from build123d import *

# Parameters (mm, degrees)
SKETCH1_W                                           = 20
SKETCH1_H                                           = 30
BOSS_EXTRUDE1_DEPTH                                 = 3
CSK_FOR_M3_COUNTERSUNK_FLAT_HEAD_SCREW1_D           = 3.6
CSK_FOR_M3_COUNTERSUNK_FLAT_HEAD_SCREW1_DEPTH       = 20
CSK_FOR_M3_COUNTERSUNK_FLAT_HEAD_SCREW1_CSINK_D     = 6.9
CSK_FOR_M3_COUNTERSUNK_FLAT_HEAD_SCREW1_CSINK_ANGLE = 90
CSK_FOR_M3_COUNTERSUNK_FLAT_HEAD_SCREW1_TIP         = 1.081549114
SKETCH4_W                                           = 8
SKETCH4_H                                           = 6
BOSS_EXTRUDE2_DEPTH                                 = 15.2
SKETCH5_W                                           = 3
SKETCH5_H                                           = 6
BOSS_EXTRUDE3_DEPTH                                 = 10
FILLET2_R                                           = 0.5
CUT_EXTRUDE1_DEPTH                                  = 4
FILLET3_R                                           = 0.5


with BuildPart() as part:
    # Sketch1 → Boss-Extrude1 (new body)
    with BuildSketch(Plane.XY):
        Rectangle(SKETCH1_W, SKETCH1_H)
    extrude(amount=BOSS_EXTRUDE1_DEPTH)

    # CSK for M3 Countersunk Flat Head Screw1
    with Locations(Plane(origin=(5, 9, 3), x_dir=(1, 0, 0), z_dir=(0, 0, 1))):
        with Locations((0, 0), (0, -18)):
            CounterSinkHole(CSK_FOR_M3_COUNTERSUNK_FLAT_HEAD_SCREW1_D / 2, CSK_FOR_M3_COUNTERSUNK_FLAT_HEAD_SCREW1_CSINK_D / 2, depth=CSK_FOR_M3_COUNTERSUNK_FLAT_HEAD_SCREW1_DEPTH, counter_sink_angle=CSK_FOR_M3_COUNTERSUNK_FLAT_HEAD_SCREW1_CSINK_ANGLE)
            with Locations((0, 0, -(CSK_FOR_M3_COUNTERSUNK_FLAT_HEAD_SCREW1_DEPTH + CSK_FOR_M3_COUNTERSUNK_FLAT_HEAD_SCREW1_TIP / 2))):  # 118° drill point
                Cone(0, CSK_FOR_M3_COUNTERSUNK_FLAT_HEAD_SCREW1_D / 2, CSK_FOR_M3_COUNTERSUNK_FLAT_HEAD_SCREW1_TIP, mode=Mode.SUBTRACT)

    # Sketch4 → Boss-Extrude2 (add)
    with BuildSketch(Plane.XY.offset(3)):
        with Locations((3, 0.108485118)):
            Rectangle(SKETCH4_W, SKETCH4_H)
    extrude(amount=BOSS_EXTRUDE2_DEPTH)

    # Sketch5 → Boss-Extrude3 (add)
    with BuildSketch(Plane.ZY.offset(1)):
        with Locations((16.7, 0.108485118)):
            Rectangle(SKETCH5_W, SKETCH5_H)
    extrude(amount=BOSS_EXTRUDE3_DEPTH)

    # Fillet2
    fillet2_edges = [part.edges().sort_by_distance(p)[0] for p in [
        (10, 0, 3),
        (0, 15, 3),
        (7, -2.891514882, 10.6),
        (7, 3.108485118, 10.6),
        (-2, -2.891514882, 18.2),
        (7, 0.108485118, 18.2),
        (-2, 3.108485118, 18.2),
        (-1, 3.108485118, 9.1),
        (-10, 0, 3),
        (-1, -2.891514882, 9.1),
        (-6, 3.108485118, 15.2),
        (-6, -2.891514882, 15.2),
        (0, 15, 0),
        (10, 0, 0),
        (0, -15, 0),
        (-10, 0, 0),
        (0, -15, 3),
    ]]
    fillet(fillet2_edges, radius=FILLET2_R)

    # Sketch6 → Cut-Extrude1 (cut, through all)
    with BuildSketch(Plane.XY.offset(3)):
        Polygon((-0.377386615, -7.652187056), (0.53847877, -7.652187056), (0.53847877, -12.027988338), (-6.483155845, -8.750907509), (-6.483155845, -11.926225518), (-7.39902123, -11.926225518), (-7.39902123, -7.346898595), (-0.377386615, -10.625569468), align=None)
    extrude(amount=-CUT_EXTRUDE1_DEPTH, mode=Mode.SUBTRACT)

    # Fillet3
    fillet3_edges = [part.edges().sort_by_distance(p)[0] for p in [
        (-11, -2.891514882, 16.7),
        (-11, 0.108485118, 15.2),
        (-11, 0.108485118, 18.2),
        (-11, 3.108485118, 16.7),
        (-11, 2.962038509, 15.346446609),
        (-11, 2.962038509, 18.053553391),
        (-11, -2.745068272, 18.053553391),
        (-11, -2.745068272, 15.346446609),
    ]]
    fillet(fillet3_edges, radius=FILLET3_R)


solid = part.part
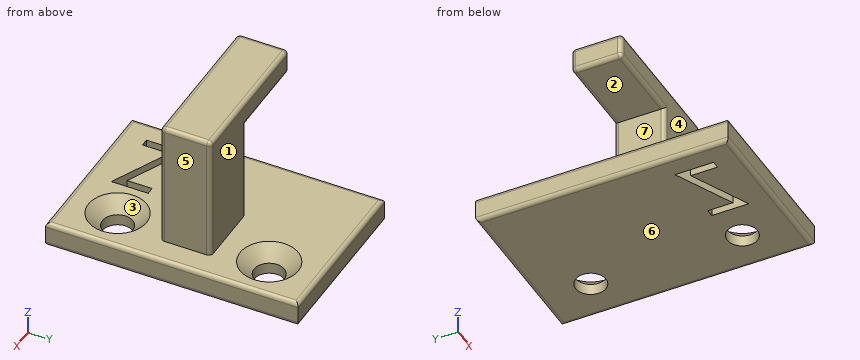
Check sheet for the modelled part. Datum: model origin and axes. Units: mm. Face numbers are marked on the shaded views. A direction names the side the tool comes from. Give positions to 0.01 mm unless a question says otherwise; leave off trailing zeros. Write each loop counter-clockwise with the first axis right and the second up, starting at its lowest first coordinate (ties: lowest second). Pieces come first, ordered by that corner, then holes. Notation, with made-up numbers: M 26,-22 L 85,-22 A25 cw 85,-2 Z; hole C 14.5,36 d9. An arc over 180 degrees is marked long. Use one line per item in the form item = value.
(1) Section check D-D on y = -3.5. Record the boundary of the cut face in (x, z).
Answer block:
outline = M -10,0.5 A0.5 ccw -9.5,0 L 9.5,0 A0.5 ccw 10,0.5 L 10,2.5 A0.5 ccw 9.5,3 L -9.5,3 A0.5 ccw -10,2.5 Z
(2) Material ranges on line 1 along Y through (x, z) = (5, 0.5); line 2 along Z through (x, y) = (-2, -0.25); line 3 along X through (y, z) = (-9, 0.75), recorded low to high.
Answer block:
line_1 = -15 to -10.8, -7.2 to 7.2, 10.8 to 15
line_2 = 0 to 3, 15.2 to 18.2
line_3 = -10 to -7.4, -6.48 to -5.95, -3.86 to -0.38, 0.54 to 3.2, 6.8 to 10
(3) Depth check by flat-ended pin: P1, Ø4, axis at y = -2, z = 16, coming from the +X side; P2, Ø6, axis at x = 5, y = 9, coming from the -Z side; P3, Ø1, axis at y = 3.5, z = 2, coming from the -X side; P4, Ø4, axis at x = 0, z = 16, coming from the -Y side. Enter the tip coordinate at first touch or a pass-through.
Answer block:
P1 = 7
P2 = 0
P3 = -10
P4 = -2.89
(4) Tool access check on the marked faces 4, 5, 6 and 7. Record the directions out of +Z, -Z, +X, -X, +Y, -Y that give a thin tool (end or side, any length) a straight path to the whole face; none if there is none.
Answer block:
face_4 = +Z, +X, -X, -Y
face_5 = +Z, +X, +Y, -Y
face_6 = -Z, +X, -X, +Y, -Y
face_7 = -X, +Y, -Y
(5) Section check A-A on x = 5. Record the boundary of the cut face in (y, z).
Answer block:
outline = M -15,0.5 A0.5 ccw -14.5,0 L -10.8,0 L -10.8,1.35 L -12.45,3 L -14.5,3 A0.5 ccw -15,2.5 Z; M -7.2,0 L 7.2,0 L 7.2,1.35 L 5.55,3 L 3.11,3 L 3.11,17.7 A0.5 ccw 2.61,18.2 L -2.39,18.2 A0.5 ccw -2.89,17.7 L -2.89,3 L -5.55,3 L -7.2,1.35 Z; M 10.8,0 L 14.5,0 A0.5 ccw 15,0.5 L 15,2.5 A0.5 ccw 14.5,3 L 12.45,3 L 10.8,1.35 Z
(6) Section check C-C on z = 17. Record the boundary of the cut face in (x, y).
Answer block:
outline = M -11,-2.39 A0.5 ccw -10.5,-2.89 L 6.5,-2.89 A0.5 ccw 7,-2.39 L 7,2.61 A0.5 ccw 6.5,3.11 L -10.5,3.11 A0.5 ccw -11,2.61 Z
(7) Section check B-B on y = 9. Record the boundary of the cut face in (x, z), plus the area to 3 significant figures.
Answer block:
outline = M -10,0.5 A0.5 ccw -9.5,0 L 3.2,0 L 3.2,1.35 L 1.55,3 L -9.5,3 A0.5 ccw -10,2.5 Z; M 6.8,0 L 9.5,0 A0.5 ccw 10,0.5 L 10,2.5 A0.5 ccw 9.5,3 L 8.45,3 L 6.8,1.35 Z
area = 46.3 mm2
(8) Draft check along Y on the marked faces 1, 2 and 3. Enter one of: pulls with the +Y half, pulls with the -Y half, needs draft (parallel to the pull), parting line crosses it, or undercut.
Answer block:
face_1 = pulls with the +Y half
face_2 = needs draft
face_3 = undercut
